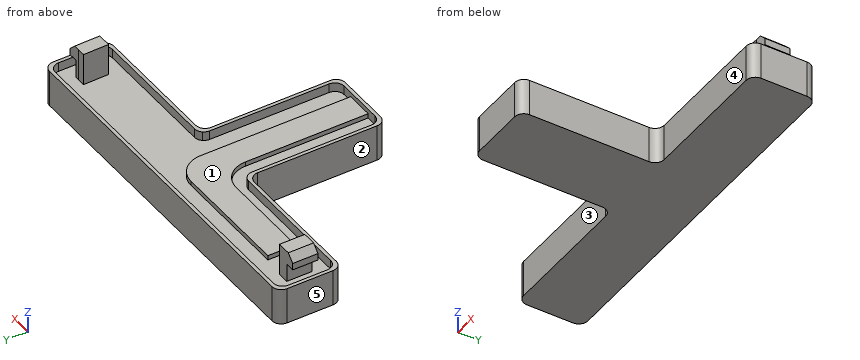
```python
from build123d import *

# Parameters (mm, degrees)
F1_DEPTH  = 6
F3_DEPTH  = 1
F5_DEPTH  = 7
F7_DEPTH  = 2
F8_W      = 2
F8_H      = 4
F9_DEPTH  = 6
F10_W     = 2
F10_H     = 4
F11_DEPTH = 6


with BuildPart() as f1:
    # F0 (on Top) → F1 (new body)
    with BuildSketch(Plane.XY):
        with BuildLine():
            Line((-35, 0), (-12, 0))
            Line((-12, 0), (-10, 0))
            ThreePointArc((-10, 0), (-8.5857864376, -0.5857864376), (-8, -2))
            Line((-8, -2), (-8, -28))
            ThreePointArc((-8, -28), (-7.4142135624, -29.4142135624), (-6, -30))
            Line((-6, -30), (0, -30))
            Line((0, -30), (6, -30))
            ThreePointArc((6, -30), (7.4142135624, -29.4142135624), (8, -28))
            Line((8, -28), (8, -2))
            ThreePointArc((8, -2), (8.5857864376, -0.5857864376), (10, 0))
            Line((10, 0), (35, 0))
            ThreePointArc((35, 0), (36.4142135624, 0.5857864376), (37, 2))
            Line((37, 2), (37, 12))
            ThreePointArc((37, 12), (36.4142135624, 13.4142135624), (35, 14))
            Line((35, 14), (-35, 14))
            ThreePointArc((-35, 14), (-36.4142135624, 13.4142135624), (-37, 12))
            Line((-37, 12), (-37, 2))
            ThreePointArc((-37, 2), (-36.4142135624, 0.5857864376), (-35, 0))
        make_face()
        with BuildLine():
            Line((-38, 0), (-35, 0))
            ThreePointArc((-35, 0), (-36.4142135624, 0.5857864376), (-37, 2))
            Line((-37, 2), (-37, 12))
            ThreePointArc((-37, 12), (-36.4142135624, 13.4142135624), (-35, 14))
            Line((-35, 14), (-38, 14))
            ThreePointArc((-38, 14), (-39.4142135624, 13.4142135624), (-40, 12))
            Line((-40, 12), (-40, 2))
            ThreePointArc((-40, 2), (-39.4142135624, 0.5857864376), (-38, 0))
        make_face()
        with BuildLine():
            Line((38, 14), (35, 14))
            ThreePointArc((35, 14), (36.4142135624, 13.4142135624), (37, 12))
            Line((37, 12), (37, 2))
            ThreePointArc((37, 2), (36.4142135624, 0.5857864376), (35, 0))
            Line((35, 0), (37, 0))
            Line((37, 0), (38, 0))
            ThreePointArc((38, 0), (39.4142135624, 0.5857864376), (40, 2))
            Line((40, 2), (40, 12))
            ThreePointArc((40, 12), (39.4142135624, 13.4142135624), (38, 14))
        make_face()
    extrude(amount=F1_DEPTH)

    # F2 (on face) → F3 (join)
    with BuildSketch(Plane.XY.offset(6)):
        with BuildLine():
            Line((-3, -2.5), (-3, -30))
            Line((-3, -30), (3, -30))
            Line((3, -30), (3, 3.5))
            ThreePointArc((3, 3.5), (1.3890872965, 7.3890872965), (-2.5, 9))
            Line((-2.5, 9), (-28.75, 9))
            Line((-28.75, 9), (-28.75, 3))
            Line((-28.75, 3), (-8.5, 3))
            ThreePointArc((-8.5, 3), (-8.2371364782, 2.9937148423), (-7.9748737342, 2.9748737342))
            ThreePointArc((-7.9748737342, 2.9748737342), (-4.4294844023, 1.1987704401), (-3, -2.5))
        make_face()
    extrude(amount=F3_DEPTH)

    # F4 (on face) → F5 (join)
    with BuildSketch(Plane.XY.offset(6)):
        Polygon((35.2363081181, 4), (38.0360990062, 4.034219625), (37.9688818856, 9.5338088696), (35.1690909975, 9.4995892445), (33.4692179582, 9.4788130436), (33.5364350788, 3.9792237991), align=None)
        Polygon((-38, 9.5), (-38, 4), (-35.2, 4), (-33.5, 4), (-33.5, 9.5), align=None)
    extrude(amount=F5_DEPTH)

    # F6 (on face) → F7 (join)
    with BuildSketch(Plane.XY.offset(6)):
        with BuildLine():
            Line((-6, -30), (0, -30))
            Line((0, -30), (6, -30))
            ThreePointArc((6, -30), (7.4142135624, -29.4142135624), (8, -28))
            Line((8, -28), (8, -2))
            ThreePointArc((8, -2), (8.5857864376, -0.5857864376), (10, 0))
            Line((10, 0), (38, 0))
            ThreePointArc((38, 0), (39.4142135624, 0.5857864376), (40, 2))
            Line((40, 2), (40, 12))
            ThreePointArc((40, 12), (39.4142135624, 13.4142135624), (38, 14))
            Line((38, 14), (-38, 14))
            ThreePointArc((-38, 14), (-39.4142135624, 13.4142135624), (-40, 12))
            Line((-40, 12), (-40, 2))
            ThreePointArc((-40, 2), (-39.4142135624, 0.5857864376), (-38, 0))
            Line((-38, 0), (-10, 0))
            ThreePointArc((-10, 0), (-8.5857864376, -0.5857864376), (-8, -2))
            Line((-8, -2), (-8, -28))
            ThreePointArc((-8, -28), (-7.4142135624, -29.4142135624), (-6, -30))
        make_face()
        with BuildLine():
            Line((5.25, -29.25), (0, -29.25))
            Line((0, -29.25), (-5.25, -29.25))
            ThreePointArc((-5.25, -29.25), (-6.6642135624, -28.6642135624), (-7.25, -27.25))
            Line((-7.25, -27.25), (-7.25, -16.2867717445))
            Line((-7.25, -16.2867717445), (-7.25, -1.25))
            ThreePointArc((-7.25, -1.25), (-7.8357864376, 0.1642135624), (-9.25, 0.75))
            Line((-9.25, 0.75), (-28.4743793309, 0.75))
            Line((-28.4743793309, 0.75), (-37.25, 0.75))
            ThreePointArc((-37.25, 0.75), (-38.6642135624, 1.3357864376), (-39.25, 2.75))
            Line((-39.25, 2.75), (-39.25, 11.25))
            ThreePointArc((-39.25, 11.25), (-38.6642135624, 12.6642135624), (-37.25, 13.25))
            Line((-37.25, 13.25), (23.7047821283, 13.25))
            Line((23.7047821283, 13.25), (37.25, 13.25))
            ThreePointArc((37.25, 13.25), (38.6642135624, 12.6642135624), (39.25, 11.25))
            Line((39.25, 11.25), (39.25, 2.75))
            ThreePointArc((39.25, 2.75), (38.6642135624, 1.3357864376), (37.25, 0.75))
            Line((37.25, 0.75), (9.25, 0.75))
            ThreePointArc((9.25, 0.75), (8.3839745962, 0.5527756377), (7.6887505004, 0))
            ThreePointArc((7.6887505004, 0), (7.3628726859, -0.5876175573), (7.25, -1.25))
            Line((7.25, -1.25), (7.25, -27.25))
            ThreePointArc((7.25, -27.25), (6.6642135624, -28.6642135624), (5.25, -29.25))
        make_face(mode=Mode.SUBTRACT)
    extrude(amount=F7_DEPTH)

    # F8 (on face) → F9 (cut)
    with BuildSketch(Plane(origin=(-0.0436186312, 3.5688014166, 0), x_dir=(0.9999253172, 0.0122212947, 0), z_dir=(0.0122212947, -0.9999253172, 0))):
        Polygon((38.0825617502, 13), (36.5825617502, 13), (38.0825617502, 11.5), align=None)
        with Locations((37.0825617502, 8)):
            Rectangle(F8_W, F8_H)
    extrude(amount=-F9_DEPTH, mode=Mode.SUBTRACT)

    # F10 (on face) → F11 (cut)
    with BuildSketch(Plane.XZ.offset(-4)):
        with Locations((-37, 8)):
            Rectangle(F10_W, F10_H)
        Polygon((-38, 11.5), (-36.5, 13), (-38, 13), align=None)
    extrude(amount=-F11_DEPTH, mode=Mode.SUBTRACT)


solid = f1.part
```
Read the model definition and answer for the solid it produces. Units are mm, in the model's axes. Face numbers are marked on the shaded views. A direction names the side the tool comes from. Give positions to 0.01 mm unless a question says otherwise; leave off trailing zeros. Order: outer loops, then holes, each group sorted by start corner. A loop starts at its lowest first (then second) coordinate and runs counter-clockwise, first axis right, second up. Notation, with made-up numbers: (69.25, 84) -> (82.25, 84) arc R18 ccw to (82.25, 99) -> close; hole circle Ø10 at (85, 50.25). An arc over 180 degrees is marked (long way). One line per item, written item: value. Start each with the question number.
(1) A tool of negligible diameter and unlimited length cuts with its end or side. For the marked faces 4 and 5, from which of +Z, -Z, +X, -X, +Y, -Y can it reach the whole face along a straight path? Write none if from no direction.
(2) The part is cut by section D-D (z = 1.5). Determine the outline of the cut face in (x, y).
(3) The part is cut by section C-C (y = -11.5). Determine the outline of the cut face in (x, z).
(4) The part is cut by section B-B (x = 21.5). Determine the outline of the cut face in (y, z), and give its area (3 significant figures).
(5) Flat-ended cylindrical pins translate along their axes: P1, Ø22, axis at x = 14, y = -12.5, coming from the +Z side; P2, Ø4, axis at y = -4, z = 2.5, coming from the -X side; P3, Ø5, axis at x = -17.5, z = 9, coming from the -Y side. Find the tip coordinate at first contact, or state that the pin passes through.
(6) Straight lines are drawn through the part: L1, parallel to X at y = -19.5, z = 7.75; L2, parallel to Z at x = 7, y = -14; L3, parallel to Y at x = 15, z = 0.75. For each, find the intervals that lie inside material, in ascending order.
(7) The part is cut by section A-A (z = 9). Determine the outline of the cut face in (x, y).
(8) For a pull along X with two mould halves and no side action, classify the marked faces 1, 2 and 3 as released by +X, released by -X, zero draft, split by the parting line, or undercut.
Taken from the geometry:
1. face 4: +Z, -Z, +X, -Y
1. face 5: +Z, -Z, -X, +Y, -Y
2. outline: (-40, 2) arc R2 ccw to (-38, 0) -> (-10, 0) arc R2 cw to (-8, -2) -> (-8, -28) arc R2 ccw to (-6, -30) -> (6, -30) arc R2 ccw to (8, -28) -> (8, -2) arc R2 cw to (10, 0) -> (38, 0) arc R2 ccw to (40, 2) -> (40, 12) arc R2 ccw to (38, 14) -> (-38, 14) arc R2 ccw to (-40, 12) -> close
3. outline: (-8, 0) -> (8, 0) -> (8, 8) -> (7.25, 8) -> (7.25, 6) -> (3, 6) -> (3, 7) -> (-3, 7) -> (-3, 6) -> (-7.25, 6) -> (-7.25, 8) -> (-8, 8) -> close
4. outline: (0, 0) -> (14, 0) -> (14, 8) -> (13.25, 8) -> (13.25, 6) -> (0.75, 6) -> (0.75, 8) -> (0, 8) -> close
4. area: 87.0 mm^2
5. P1: z = 8
5. P2: x = -8
5. P3: y = 0
6. L1: -8 to -7.25, 7.25 to 8
6. L2: 0 to 6
6. L3: 0 to 14
7. outline: (-36, 4) -> (-33.5, 4) -> (-33.5, 9.5) -> (-36, 9.5) -> close; (33.47, 9.48) -> (33.54, 3.98) -> (36.04, 4.01) -> (35.97, 9.51) -> close
8. face 1: undercut
8. face 2: released by -X
8. face 3: zero draft
